from build123d import *

# Parameters (mm, degrees)
EXTRUDE_1_DEPTH     = 5
SKETCH_2_W          = 5
SKETCH_2_H          = 25
EXTRUDE_2_DEPTH     = 10
EXTRUDE_3_DEPTH     = 43
EXTRUDE_4_DEPTH     = 10
CUT_EXTRUDE_1_DEPTH = 58
EXTRUDE_5_DEPTH     = 7
EXTRUDE_6_DEPTH     = 7
EXTRUDE_7_DEPTH     = 10
EXTRUDE_8_DEPTH     = 72
SKETCH_10_W         = 10
SKETCH_10_H         = 20.288176
EXTRUDE_9_DEPTH     = 5.9
FILLET_START        = -61
FILLET_1_DEPTH      = 74
FILLET_START_2      = -53.20464
FILLET_1_2_DEPTH    = 57.6
FILLET_START_3      = -60
FILLET_1_3_DEPTH    = 10
FILLET_START_4      = 2
FILLET_1_4_DEPTH    = 10
SKETCH_11_W         = 20.288176
SKETCH_11_H         = 3
EXTRUDE_10_DEPTH    = 5
SKETCH_12_R         = 1.6
CUT_EXTRUDE_2_DEPTH = 3
FILLET_3_R          = 1
SKETCH_13_W         = 15
SKETCH_13_H         = 3
EXTRUDE_11_DEPTH    = 2
CUT_EXTRUDE_3_REACH = 83.122
SKETCH_14_W         = 20
SKETCH_14_H         = 10
EXTRUDE_12_DEPTH    = 10
EXTRUDE_START       = 2
EXTRUDE_13_DEPTH    = 15
SKETCH_20_W         = 18
SKETCH_20_H         = 18
CUT_EXTRUDE_5_DEPTH = 98.660914
FILLET_7_R          = 5
CUT_EXTRUDE_6_DEPTH = 98.660914
FILLET_8_R          = 5
FILLET_9_R          = 5
SKETCH_22_W         = 5
SKETCH_22_H         = 18
CUT_EXTRUDE_7_DEPTH = 98.660914
FILLET_10_R         = 3
CUT_EXTRUDE_8_REACH = 98.904
SKETCH_23_R         = 1.6


with BuildPart() as part:
    # 草图1 → 凸台-拉伸1 (new body)
    with BuildSketch(Plane(origin=(0, 0, 0), x_dir=(0, 0, -1), z_dir=(1, 0, 0))):
        Polygon((0, 0), (11.868353, 9.172906), (-3.419823, 28.953494), (-15.288176, 19.780588), align=None)
    extrude(amount=EXTRUDE_1_DEPTH)

    # 草图2 → 凸台-拉伸2 (add)
    with BuildSketch(Plane(origin=(0, 0, 0), x_dir=(1, 0, 0), z_dir=(0, -0.6115270401858328, 0.7912235329674888))):
        with Locations((2.5, 12.5)):
            Rectangle(SKETCH_2_W, SKETCH_2_H)
    extrude(amount=EXTRUDE_2_DEPTH)

    # 草图3 → 凸台-拉伸3 (add)
    with BuildSketch(Plane.ZY):
        Polygon((23.200411, 13.665318), (15.288176, 19.780588), (0, 0), (7.912235, -6.11527), align=None)
    extrude(amount=EXTRUDE_3_DEPTH)

    # 草图4 → 凸台-拉伸4 (add)
    with BuildSketch(Plane.ZY.offset(43)):
        Polygon((15.288176, 19.780588), (3.419823, 28.953494), (-11.868353, 9.172906), (0, 0), (7.912235, -6.11527), (23.200411, 13.665318), align=None)
    extrude(amount=EXTRUDE_4_DEPTH)

    # 草图5 → 切除-拉伸1 (cut)
    with BuildSketch(Plane.ZY.offset(53)):
        Polygon((15.288176, 19.780588), (3.419823, 28.953494), (-11.868353, 9.172906), (0, 0), align=None)
    extrude(amount=-CUT_EXTRUDE_1_DEPTH, mode=Mode.SUBTRACT)

    # 草图6 → 凸台-拉伸5 (add)
    with BuildSketch(Plane.ZY.offset(53)):
        Polygon((15.288176, 19.780588), (0, 0), (7.912235, -6.11527), (23.200411, 13.665318), align=None)
    extrude(amount=EXTRUDE_5_DEPTH)

    # 草图7 → 凸台-拉伸6 (add)
    with BuildSketch(Plane(origin=(5, 0, 0), x_dir=(0, 0, -1), z_dir=(1, 0, 0))):
        Polygon((0, 0), (-15.288176, 19.780588), (-23.200411, 13.665318), (-7.912235, -6.11527), align=None)
    extrude(amount=EXTRUDE_6_DEPTH)

    # 草图8 → 凸台-拉伸7 (add)
    with BuildSketch(Plane(origin=(12, 0, 0), x_dir=(0, 0, -1), z_dir=(1, 0, 0))):
        Polygon((-23.200411, 13.665318), (-28.200411, 13.665318), (-28.200411, -24.848688), (-28.200411, -32.095582), (-7.912235, -32.095582), (-7.912235, -24.848688), (-7.912235, -6.11527), align=None)
    extrude_7 = extrude(amount=-EXTRUDE_7_DEPTH)

    # 镜向1: 凸台-拉伸7 across plane
    add(extrude_7.mirror(Plane.ZY.offset(24)))

    # 草图9 → 凸台-拉伸8 (add)
    with BuildSketch(Plane.ZY.offset(60)):
        Polygon((23.200411, 13.665318), (28.200411, 13.665318), (28.200411, 19.780588), (15.288176, 19.780588), align=None)
    extrude(amount=-EXTRUDE_8_DEPTH)

    # 草图10 → 凸台-拉伸9 (add)
    with BuildSketch(Plane.XZ.offset(32.095582)):
        with Locations((7, 18.056323)):
            Rectangle(SKETCH_10_W, SKETCH_10_H)
        with Locations((-55, 18.056323)):
            Rectangle(SKETCH_10_W, SKETCH_10_H)
    extrude(amount=EXTRUDE_9_DEPTH)

    # 圆角1: read off the stored shape, not the designer's step
    # 圆角1 outline → 圆角1 (cut)
    with BuildSketch(Plane.YZ.offset(FILLET_START)):
        with BuildLine():
            Line((19.780588, 28.200411), (16.780588, 28.200411))
            ThreePointArc((16.780588, 28.200411), (18.901909, 27.321732), (19.780588, 25.200411))
            Line((19.780588, 25.200411), (19.780588, 28.200411))
        make_face()
    extrude(amount=FILLET_1_DEPTH, mode=Mode.SUBTRACT)

    # Fillet 1 2 outline → Fillet 1 2 (add)
    with BuildSketch(Plane.YZ.offset(FILLET_START_2)):
        with BuildLine():
            ThreePointArc((13.665318, 24.673344), (13.358248, 23.351176), (12.499899, 22.299673))
            Line((12.499899, 22.299673), (13.665318, 23.200411))
            Line((13.665318, 23.200411), (13.665318, 24.673344))
        make_face()
    extrude(amount=FILLET_1_2_DEPTH)

    # Fillet 1 3 outline → Fillet 1 3 (add)
    with BuildSketch(Plane.YZ.offset(FILLET_START_3)):
        with BuildLine():
            ThreePointArc((-7.588203, 7.912235), (-6.266035, 7.605165), (-5.214532, 6.746816))
            Line((-5.214532, 6.746816), (-6.11527, 7.912235))
            Line((-6.11527, 7.912235), (-7.588203, 7.912235))
        make_face()
    extrude(amount=FILLET_1_3_DEPTH)

    # Fillet 1 4 outline → Fillet 1 4 (add)
    with BuildSketch(Plane.YZ.offset(FILLET_START_4)):
        with BuildLine():
            ThreePointArc((-7.588203, 7.912235), (-6.266035, 7.605165), (-5.214532, 6.746816))
            Line((-5.214532, 6.746816), (-6.11527, 7.912235))
            Line((-6.11527, 7.912235), (-7.588203, 7.912235))
        make_face()
    extrude(amount=FILLET_1_4_DEPTH)

    # 草图11 → 凸台-拉伸10 (add)
    with BuildSketch(Plane(origin=(12, 0, 0), x_dir=(0, 0, -1), z_dir=(1, 0, 0))):
        with Locations((-18.056323, -36.495582)):
            Rectangle(SKETCH_11_W, SKETCH_11_H)
    extrude_10 = extrude(amount=EXTRUDE_10_DEPTH)

    # 草图12 → 切除-拉伸2 (cut)
    with BuildSketch(Plane(origin=(0, -34.995582, 0), x_dir=(1, 0, 0), z_dir=(0, 1, 0))):
        with Locations((14.243648, -27.816949)):
            Circle(SKETCH_12_R)
    cut_extrude_2 = extrude(amount=-CUT_EXTRUDE_2_DEPTH, mode=Mode.SUBTRACT)

    # 镜向2: 凸台-拉伸10, 切除-拉伸2 across plane
    add(extrude_10.mirror(Plane.ZY.offset(24)))
    add(cut_extrude_2.mirror(Plane.ZY.offset(24)), mode=Mode.SUBTRACT)

    # 圆角3
    fillet_3_edges = [part.edges().sort_by_distance(p)[0] for p in [
        (-24, 0, 0),
    ]]
    fillet(fillet_3_edges, radius=FILLET_3_R)

    # 草图13 → 凸台-拉伸11 (add)
    with BuildSketch(Plane.XY.offset(28.200411)):
        with Locations((-57.5, -36.495582)):
            Rectangle(SKETCH_13_W, SKETCH_13_H)
        with Locations((9.5, -36.495582)):
            Rectangle(SKETCH_13_W, SKETCH_13_H)
    extrude(amount=EXTRUDE_11_DEPTH)

    # 草图14 → 切除-拉伸3 (cut, up to next)
    with BuildSketch(Plane(origin=(0, 0, 0), x_dir=(-1, 0, 0), z_dir=(0, 0.6115270401858329, -0.7912235329674886)), mode=Mode.PRIVATE) as cut_extrude_3_sk1:
        with Locations((24, 13)):
            Rectangle(SKETCH_14_W, SKETCH_14_H)
    cut_extrude_3_tool1 = extrude(cut_extrude_3_sk1.sketch, amount=-CUT_EXTRUDE_3_REACH, mode=Mode.PRIVATE) & part.part
    add(cut_extrude_3_tool1.solids().sort_by_distance((-24, 10.285906, 7.949852))[0], mode=Mode.SUBTRACT)

    # 草图18 → 凸台-拉伸12 (add)
    with BuildSketch(Plane(origin=(12, 0, 0), x_dir=(0, 0, -1), z_dir=(1, 0, 0))):
        with BuildLine():
            Line((-24.411336, 19.674955), (-24.411336, -37.995582))
            Line((-24.411336, -37.995582), (-46.496356, -37.995582))
            add(Edge.make_bspline(
                [(-24.411336, 19.674955), (-47.385024, -2.496577), (-46.496356, -37.995582)],
                knots=[0, 0, 0, 1, 1, 1], degree=2))
        make_face()
    extrude_12 = extrude(amount=-EXTRUDE_12_DEPTH)

    # 凸台-拉伸13: read off the stored shape, not the designer's step
    # 凸台-拉伸13 outline → 凸台-拉伸13 (add)
    with BuildSketch(Plane.YZ.offset(EXTRUDE_START)):
        with BuildLine():
            Line((-34.995582, 30.200411), (-34.995582, 46.528767))
            add(Edge.make_bspline(
                [(-34.995582, 46.528767), (-36.483492, 46.534209), (-37.995582, 46.496356)],
                knots=[0.957405, 0.957405, 0.957405, 1, 1, 1], degree=2))
            Line((-37.995582, 46.496356), (-37.995582, 30.200411))
            Line((-37.995582, 30.200411), (-34.995582, 30.200411))
        make_face()
    extrude_13 = extrude(amount=EXTRUDE_13_DEPTH)

    # 镜向3: 凸台-拉伸12, 凸台-拉伸13 across plane
    add(extrude_12.mirror(Plane.ZY.offset(24)))
    add(extrude_13.mirror(Plane.ZY.offset(24)))

    # 草图20 → 切除-拉伸5 (cut, through all)
    with BuildSketch(Plane(origin=(12, 0, 0), x_dir=(0, 0, -1), z_dir=(1, 0, 0))):
        with Locations((-22.365109, -17.186728)):
            Rectangle(SKETCH_20_W, SKETCH_20_H)
    extrude(amount=-CUT_EXTRUDE_5_DEPTH, mode=Mode.SUBTRACT)

    # 圆角7
    fillet_7_edges = [part.edges().sort_by_distance(p)[0] for p in [
        (17, -36.489537, 46.523386),
        (-65, -36.495582, 7.912235),
        (17, -36.495582, 7.912235),
        (-65, -36.489537, 46.523386),
    ]]
    fillet(fillet_7_edges, radius=FILLET_7_R - 0.0001)  # a hair under: the kernel refuses the full size

    # 草图21 → 切除-拉伸6 (cut, through all)
    with BuildSketch(Plane(origin=(12, 0, 0), x_dir=(0, 0, -1), z_dir=(1, 0, 0))):
        with BuildLine():
            Line((-28.200411, 15.747176), (-24.166999, 19.780588))
            Line((-24.166999, 19.780588), (-25.200411, 19.780588))
            ThreePointArc((-25.200411, 19.780588), (-27.321732, 18.901909), (-28.200411, 16.780588))
            Line((-28.200411, 16.780588), (-28.200411, 15.747176))
        make_face()
    extrude(amount=-CUT_EXTRUDE_6_DEPTH, mode=Mode.SUBTRACT)

    # 圆角8
    fillet_8_edges = [part.edges().sort_by_distance(p)[0] for p in [
        (-24, 19.780588, 24.166999),
    ]]
    fillet(fillet_8_edges, radius=FILLET_8_R)

    # 圆角9
    fillet_9_edges = [part.edges().sort_by_distance(p)[0] for p in [
        (-24, 19.780588, 15.288176),
    ]]
    fillet(fillet_9_edges, radius=FILLET_9_R)

    # 草图22 → 切除-拉伸7 (cut, through all)
    with BuildSketch(Plane.ZY.offset(60)):
        with Locations((33.865109, -17.186728)):
            Rectangle(SKETCH_22_W, SKETCH_22_H)
    extrude(amount=-CUT_EXTRUDE_7_DEPTH, mode=Mode.SUBTRACT)

    # 圆角10
    fillet_10_edges = [part.edges().sort_by_distance(p)[0] for p in [
        (7, -8.186728, 13.365109),
        (-55, -8.186728, 13.365109),
        (7, -26.186728, 13.365109),
        (-55, -26.186728, 13.365109),
        (7, -8.186728, 36.365109),
        (-55, -8.186728, 36.365109),
        (7, -26.186728, 36.365109),
        (-55, -26.186728, 36.365109),
    ]]
    fillet(fillet_10_edges, radius=FILLET_10_R)

    # 草图23 → 切除-拉伸8 (cut, up to next)
    with BuildSketch(Plane(origin=(0, -34.995582, 0), x_dir=(1, 0, 0), z_dir=(0, 1, 0)), mode=Mode.PRIVATE) as cut_extrude_8_sk1:
        with Locations(Location((14.243648, -27.816949, 0), (0, 0, 270))):
            Circle(SKETCH_23_R)
    cut_extrude_8_tool1 = extrude(cut_extrude_8_sk1.sketch, amount=-CUT_EXTRUDE_8_REACH, mode=Mode.PRIVATE) & part.part
    # 草图23 → 切除-拉伸8 (cut, up to next)
    with BuildSketch(Plane(origin=(0, -34.995582, 0), x_dir=(1, 0, 0), z_dir=(0, 1, 0)), mode=Mode.PRIVATE) as cut_extrude_8_sk2:
        with Locations(Location((-62.243648, -27.816949, 0), (0, 0, 270))):
            Circle(SKETCH_23_R)
    cut_extrude_8_tool2 = extrude(cut_extrude_8_sk2.sketch, amount=-CUT_EXTRUDE_8_REACH, mode=Mode.PRIVATE) & part.part
    add(cut_extrude_8_tool1.solids().sort_by_distance((14.243648, -34.995582, 27.816949))[0], mode=Mode.SUBTRACT)
    add(cut_extrude_8_tool2.solids().sort_by_distance((-62.243648, -34.995582, 27.816949))[0], mode=Mode.SUBTRACT)


solid = part.part
The model under review builds one solid part; all positions refer to its coordinate system, in mm. A direction names the side the tool comes from. Round coordinates to 2 decimals unless told otherwise and drop trailing zeros. Order: outer loops, then holes, each group sorted by start corner. A loop starts at its lowest first (then second) coordinate and runs counter-clockwise, first axis right, second up. Notation, with made-up numbers: (8.25, 62) -> (40.25, 62) arc R20 ccw to (40.25, 88) -> close; hole circle Ø1 at (62, 47). An arc over 180 degrees is marked (long way). Write item = value, one per line. Start each with the question number.
Item 1: Clearance check with flat-ended pins moving along their axes: pin 1 Ø4 at (y, z) = (8, 13.5) entering from +X; pin 2 Ø1.5 at (x, y) = (-34, 8.5) entering from -Z; pin 3 Ø8 at (x, y) = (-56.5, -16) entering from +Z; pin 4 Ø12 at (y, z) = (-20, 19.5) entering from -X. State where each tip first meets the part, or that it passes through.
Item 2: Consider section B-B on x = -13. Write out the cut boundary in (y, z).
Item 3: For line 1 along X through (y, z) = (-22.5, 10); line 2 along Y through (x, z) = (-58.5, 19.5); line 3 along X through (y, z) = (3.5, 14.5), list the stretches that pass through material, from the lowest coordinate up.
Item 4: Mouldability with a two-part tool opening along Z and no side actions: class faces 1 (the face through (-58, -37.996, 27)), 2 (the face through (-54.93, -25.331, 35.463)), 3 (the face through (-63.5, -36.47, 9.34)) as released by +Z, released by -Z, zero draft, split by the parting line, or undercut.
Item 5: Consider section C-C on y = -22. Count the separate pieces of the cut face and the enclosed holes in it, plus the area to 3 significant figures.
Item 6: For faces 4 (the face through (12, -7, 23)), 5 (the face through (-23.86, 11.227, 14.908)), 6 (the face through (-64, -34.996, 27)), 7 (the face through (-23.86, 3.315, 8.793)), 8 (the face through (7, -8.187, 25)), list the 3-axis set-ups (+Z, -Z, +X, -X, +Y, -Y) from which the entire face can be reached by the end or side of a thin tool; tool diameter is ignored.
Item 7: Consider section A-A on x = -23.5. Write out the cut boundary in (y, z).
Item 8: Consider section D-D on z = 4. Write out the cut boundary in (x, y), plus the area to 3 significant figures.
Conclusion:
q1.pin_1 = 12
q1.pin_2 = 5.99
q1.pin_3 = 45.27
q1.pin_4 = through
q2.outline = (-6.12, 7.91) -> (-0.61, 0.79) arc R1 ccw to (0.79, 0.61) -> (17.84, 13.79) arc R5 ccw to (19.78, 17.74) -> (19.78, 22.1) arc R5 ccw to (18.32, 25.63) -> (15.75, 28.2) -> (13.67, 28.2) -> (13.67, 24.67) arc R3 cw to (12.5, 22.3) -> close
q3.line_1 = -60 to -50, 2 to 12
q3.line_2 = -38 to -26.19, -8.19 to 19.78
q3.line_3 = -60 to -34, -14 to 12
q4.face_1 = zero draft
q4.face_2 = undercut
q4.face_3 = released by -Z
q5.separate_pieces = 4
q5.enclosed_holes = 0
q5.area = 294 mm2
q6.face_4 = +Z, -Z, +X, +Y
q6.face_5 = -Z
q6.face_6 = +Z, -Z, -X, +Y
q6.face_7 = +Z
q6.face_8 = +X, -X
q7.outline = (-6.12, 7.91) -> (-0.61, 0.79) arc R1 ccw to (0.79, 0.61) -> (6.33, 4.89) -> (0.21, 12.8) -> close; (8.13, 18.92) -> (14.24, 11.01) -> (17.84, 13.79) arc R5 ccw to (19.78, 17.74) -> (19.78, 22.1) arc R5 ccw to (18.32, 25.63) -> (15.75, 28.2) -> (13.67, 28.2) -> (13.67, 24.67) arc R3 cw to (12.5, 22.3) -> close
q8.outline = (-60, -3.09) -> (12, -3.09) -> (12, 5.18) -> (-60, 5.18) -> close
q8.area = 595 mm2
